Model file for the job. Use its own axes, mm. A direction names the side the tool comes from. Round coordinates to 2 decimals unless told otherwise and drop trailing zeros. Order: outer loops, then holes, each group sorted by start corner. A loop starts at its lowest first (then second) coordinate and runs counter-clockwise, first axis right, second up. Notation, with made-up numbers: M 32,-39 L 89,-39 A28 ccw 89,-19 Z; hole C -15.5,-28.5 d6. An arc over 180 degrees is marked long. Return JSON: item names as keys, results as strings. Group by question number.
Item 1: Which spindle directions (+Z, -Z, +X, -X, +Y, -Y) get a long thin tool onto all of the face, cutting with end or side? Do faces 5 (the face through (8, 0, 4)), 6 (the face through (0, -1, 2)). Say none if no direction does.
Item 2: Slice it at D-D on z = 12.5. Write the cut outline in (x, y).
Item 3: Pull direction X, two halves, no side cores. Call faces 1 (the face through (0, -2.25, 8)), 2 (the face through (6.5, -1, 6)), 3 (the face through (-8, 0, 4)), 4 (the face through (0, 0.25, 6)): pulls with the +X half, pulls with the -X half, needs draft (parallel to the pull), parting line crosses it, or undercut.
Item 4: Probe line 1 along X through (y, z) = (-0.5, 5.25); line 2 along Y through (x, z) = (4.25, 3.5); line 3 along Z through (x, y) = (2.75, 1.25). List the from-to ranges inside material, lowest first.
Item 5: Pin check, flat tip, straight feed: pin 1 Ø0.6 at (x, y) = (-3, -1) entering from +Z. Stop position of the tip, or through.
Item 6: Slice it at B-B on y = -1.1. Write the cut outline in (x, z).
Item 7: Slice it at A-A on z = 2.5. Write the cut outline in (x, y), then the cut area to 3 significant figures.
Item 8: Slice it at C-C on x = -2.25. Write the cut outline in (y, z).
from build123d import *

# Parameters (mm, degrees)
F0_W     = 16
F0_H     = 4.5
F1_DEPTH = 9
F2_W     = 13
F2_H     = 2
F3_DEPTH = 7
F4_W     = 12
F4_H     = 0.5
F5_DEPTH = 8


with BuildPart() as f1:
    # F0 (on Top) → F1 (new body)
    with BuildSketch(Plane.XY):
        Rectangle(F0_W, F0_H)
    extrude(amount=F1_DEPTH)

    # F2 (on face) → F3 (cut)
    with BuildSketch(Plane.XY.offset(9)):
        with Locations((0, -0.75)):
            Rectangle(F2_W, F2_H)
    extrude(amount=-F3_DEPTH, mode=Mode.SUBTRACT)

    # F4 (on face) → F5 (join)
    with BuildSketch(Plane.XY.offset(9)):
        with Locations((0, -2)):
            Rectangle(F4_W, F4_H)
    extrude(amount=F5_DEPTH)


solid = f1.part
Output values:
{
 "1": {"face 5": "+Z, -Z, +X, +Y, -Y", "face 6": "+Z"},
 "2": {"outline": "M -6,-2.25 L 6,-2.25 L 6,-1.75 L -6,-1.75 Z"},
 "3": {"face 1": "needs draft", "face 2": "undercut", "face 3": "pulls with the -X half", "face 4": "undercut"},
 "4": {"line 1": "-8 to -6.5, 6.5 to 8", "line 2": "-2.25 to -1.75, 0.25 to 2.25", "line 3": "0 to 9"},
 "5": {"pin 1": "z = 2"},
 "6": {"outline": "M -8,0 L 8,0 L 8,9 L 6.5,9 L 6.5,2 L -6.5,2 L -6.5,9 L -8,9 Z"},
 "7": {"outline": "M -8,-2.25 L 8,-2.25 L 8,2.25 L -8,2.25 Z; hole M -6.5,-1.75 L 6.5,-1.75 L 6.5,0.25 L -6.5,0.25 Z", "area": "46.0 mm²"},
 "8": {"outline": "M -2.25,0 L 2.25,0 L 2.25,9 L 0.25,9 L 0.25,2 L -1.75,2 L -1.75,17 L -2.25,17 Z"}
}
